```python
from build123d import *

# Parameters (mm, degrees)
PAD_DEPTH     = 3
SKETCH001_R   = 15
SKETCH001_R_2 = 10
POCKET_DEPTH  = 3.001


with BuildPart() as part:
    # Sketch → Pad (new body)
    with BuildSketch(Plane.XY):
        Polygon((0, 500), (150, 500), (150, 0), (0, 0), (0, 250), align=None)
    extrude(amount=PAD_DEPTH)

    # Sketch001 (on Face7 of Pad) → Pocket (cut, through all)
    with BuildSketch(Plane.XY.offset(3)):
        with Locations((31.579084, 67.777323)):
            Circle(SKETCH001_R)
        with Locations((50.054292, 99.777323)):
            Circle(SKETCH001_R)
        with Locations((68.529501, 131.777323)):
            Circle(SKETCH001_R)
        with Locations((50.054292, 163.777323)):
            Circle(SKETCH001_R)
        with Locations((71, 246.635039)):
            Circle(SKETCH001_R_2)
        with Locations((68.529501, 67.777323)):
            Circle(SKETCH001_R)
        with Locations((88.15941, 101.777323)):
            Circle(SKETCH001_R)
        with Locations((88.15941, 163.777323)):
            Circle(SKETCH001_R)
        with Locations((53.441466, 300.257294)):
            Circle(SKETCH001_R)
        with Locations((71.916674, 332.257294)):
            Circle(SKETCH001_R)
        with Locations((90.391883, 364.257294)):
            Circle(SKETCH001_R)
        with Locations((71.916674, 396.257294)):
            Circle(SKETCH001_R)
        with Locations((71, 458)):
            Circle(SKETCH001_R_2)
        with Locations((90.391883, 300.257294)):
            Circle(SKETCH001_R)
        with Locations((110.021792, 334.257294)):
            Circle(SKETCH001_R)
        with Locations((110.021792, 396.257294)):
            Circle(SKETCH001_R)
    extrude(amount=-POCKET_DEPTH, mode=Mode.SUBTRACT)


solid = part.part
```
Source: CAD feature listing. Evaluate the final solid. Frame: model axes, mm. Coordinates: 2 decimals unless noted, no trailing zeros. Loops run counter-clockwise (first coordinate to the right, second up) from the corner with the lowest first, then second, coordinate; pieces in that order, holes last. Notation, with made-up numbers: (39.25, 51.25) -> (54.25, 51.25) arc R19 cw to (54.25, 61.25) -> close; hole circle Ø6 at (-11.5, 3.25). An arc over 180 degrees is marked (long way). One line per item, written item: value. Start each with the question number.
Q1. Section query B-B, the plane z = 1.9. Give the number of separate pieces and of enclosed holes in the cut face, and give its area (3 significant figures).
Q2. Section query A-A, the plane y = 458. Return the cut outline in (x, z).
Q3. Contact query for a flat-ended pin moving along its axis: P1, Ø18, axis at x = 110.02, y = 396.26, coming from the +Z side. Output: stop coordinate, or through.
Q4. Line query: line 1 along X through (y, z) = (391, 2.35); line 2 along X through (y, z) = (329, 2.3); line 3 along Y through (x, z) = (49.5, 0.8). Output: solid intervals per line, ascending.
Q5. Section query C-C, the plane y = 373.5. Return the cut outline in (x, z).
Q6. Mould query, pull axis Y, two halves, no side actions, for faces 1 (the face through (69.698, 467.915, 1.521)), 2 (the face through (93, 254, 0)). Classes: pulls with the +Y half, pulls with the -Y half, needs draft (parallel to the pull), parting line crosses it, or undercut.
Results:
1. separate pieces: 1
1. enclosed holes: 16
1. area: 64,500 mm^2
2. outline: (0, 0) -> (61, 0) -> (61, 3) -> (0, 3) -> close; (81, 0) -> (150, 0) -> (150, 3) -> (81, 3) -> close
3. P1: through
4. line 1: 0 to 57.87, 85.97 to 95.97, 124.07 to 150
4. line 2: 0 to 57.27, 86.56 to 95.97, 124.07 to 150
4. line 3: 0 to 84.79, 114.77 to 148.79, 178.77 to 285.78, 314.73 to 500
5. outline: (0, 0) -> (78.58, 0) -> (78.58, 3) -> (0, 3) -> close; (102.21, 0) -> (150, 0) -> (150, 3) -> (102.21, 3) -> close
6. face 1: undercut
6. face 2: needs draft
